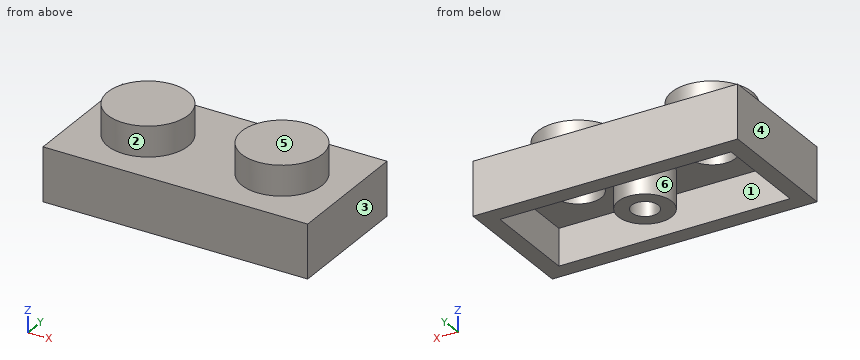
```python
from build123d import *

# Parameters (mm, degrees)
F0_W     = 15.8
F0_H     = 7.8
F1_DEPTH = 3.2
F2_R     = 2.4
F3_DEPTH = 1.8
F4_T     = -1
F5_R     = 1.6
F5_R_2   = 0.8
F6_DEPTH = 2.2


with BuildPart() as f1:
    # F0 (on Top) → F1 (new body)
    with BuildSketch(Plane.XY):
        Rectangle(F0_W, F0_H)
    extrude(amount=F1_DEPTH)

    # F2 (on face) → F3 (join)
    with BuildSketch(Plane.XY.offset(3.2)):
        with Locations((-4, 0)):
            Circle(F2_R)
        with Locations((4, 0)):
            Circle(F2_R)
    extrude(amount=F3_DEPTH)

    # F4
    f4_openings = [f1.faces().sort_by_distance(p)[0] for p in [
        (0, 0, 0),
    ]]
    offset(amount=F4_T, openings=f4_openings, kind=Kind.INTERSECTION)

    # F5 (on face) → F6 (join, through all)
    with BuildSketch(Plane(origin=(0, 0, 2.2), x_dir=(1, 0, 0), z_dir=(0, 0, -1))):
        Circle(F5_R)
        Circle(F5_R_2, mode=Mode.SUBTRACT)
    extrude(amount=F6_DEPTH)


solid = f1.part
```
Part model, mm, in its own coordinate system. Face numbers are marked on the shaded views. A direction names the side the tool comes from. Round coordinates to 2 decimals unless told otherwise and drop trailing zeros. Write each loop counter-clockwise with the first axis right and the second up, starting at its lowest first coordinate (ties: lowest second). Pieces come first, ordered by that corner, then holes. Notation, with made-up numbers: (28.25, 45) -> (47.25, 45) arc R25 cw to (47.25, 57) -> close; hole circle Ø8 at (37, 2). An arc over 180 degrees is marked (long way). Return JSON: item names as keys, results as strings. Group by question number.
Q1. Saw through at C-C on z = 4.15. Write the cut outline in (x, y).
Q2. Probe L1, parallel to X at y = 0, z = 0.75; L2, parallel to Y at x = -4, z = 3.15; L3, parallel to X at y = 0, z = 3.15. List the from-to ranges inside material, lowest first. Write a range as [from, to].
Q3. Saw through at A-A on z = 1.7. Write the cut outline in (x, y), plus the area to 3 significant figures.
Q4. Pin check, flat tips, straight feed: pin 1 (3 mm diameter, centred on x = -4, y = 0.5, fed in from -Z); pin 2 (2.5 mm diameter, centred on x = 0, y = 0, fed in from +Z); pin 3 (3 mm diameter, centred on x = 4, y = 3, fed in from -Z); pin 4 (2.5 mm diameter, centred on x = 4, y = 0, fed in from -Z). Stop position of each tip, or through.
Q5. Which spindle directions (+Z, -Z, +X, -X, +Y, -Y) get a long thin tool onto all of the face, cutting with end or side? Do the marked faces 1, 2 and 3. Say none if no direction does.
Q6. Saw through at B-B on x = 0. Write the cut outline in (y, z).
Q7. Mould opens along X. For the marked faces 4, 5 and 6 say: pulls with the +X half, pulls with the -X half, needs draft (parallel to the pull), parting line crosses it, or undercut.
Answer:
{
 "1": {"outline": "circle Ø4.8 at (-4, 0); circle Ø4.8 at (4, 0)"},
 "2": {"L1": "[-7.9, -6.9], [-1.6, -0.8], [0.8, 1.6], [6.9, 7.9]", "L2": "[-3.9, -1.4], [1.4, 3.9]", "L3": "[-7.9, -5.4], [-2.6, 2.6], [5.4, 7.9]"},
 "3": {"outline": "(-7.9, -3.9) -> (7.9, -3.9) -> (7.9, 3.9) -> (-7.9, 3.9) -> close; circle Ø3.2 at (0, 0); hole (-6.9, -2.9) -> (6.9, -2.9) -> (6.9, 2.9) -> (-6.9, 2.9) -> close; hole circle Ø1.6 at (0, 0)", "area": "49.2 mm2"},
 "4": {"pin 1": "z = 2.2", "pin 2": "z = 3.2", "pin 3": "z = 0", "pin 4": "z = 4"},
 "5": {"face 1": "-Z", "face 2": "+Z", "face 3": "+Z, -Z, +X, +Y, -Y"},
 "6": {"outline": "(-3.9, 0) -> (-2.9, 0) -> (-2.9, 2.2) -> (-1.6, 2.2) -> (-1.6, 0) -> (-0.8, 0) -> (-0.8, 2.2) -> (0.8, 2.2) -> (0.8, 0) -> (1.6, 0) -> (1.6, 2.2) -> (2.9, 2.2) -> (2.9, 0) -> (3.9, 0) -> (3.9, 3.2) -> (-3.9, 3.2) -> close"},
 "7": {"face 4": "pulls with the -X half", "face 5": "needs draft", "face 6": "undercut"}
}
